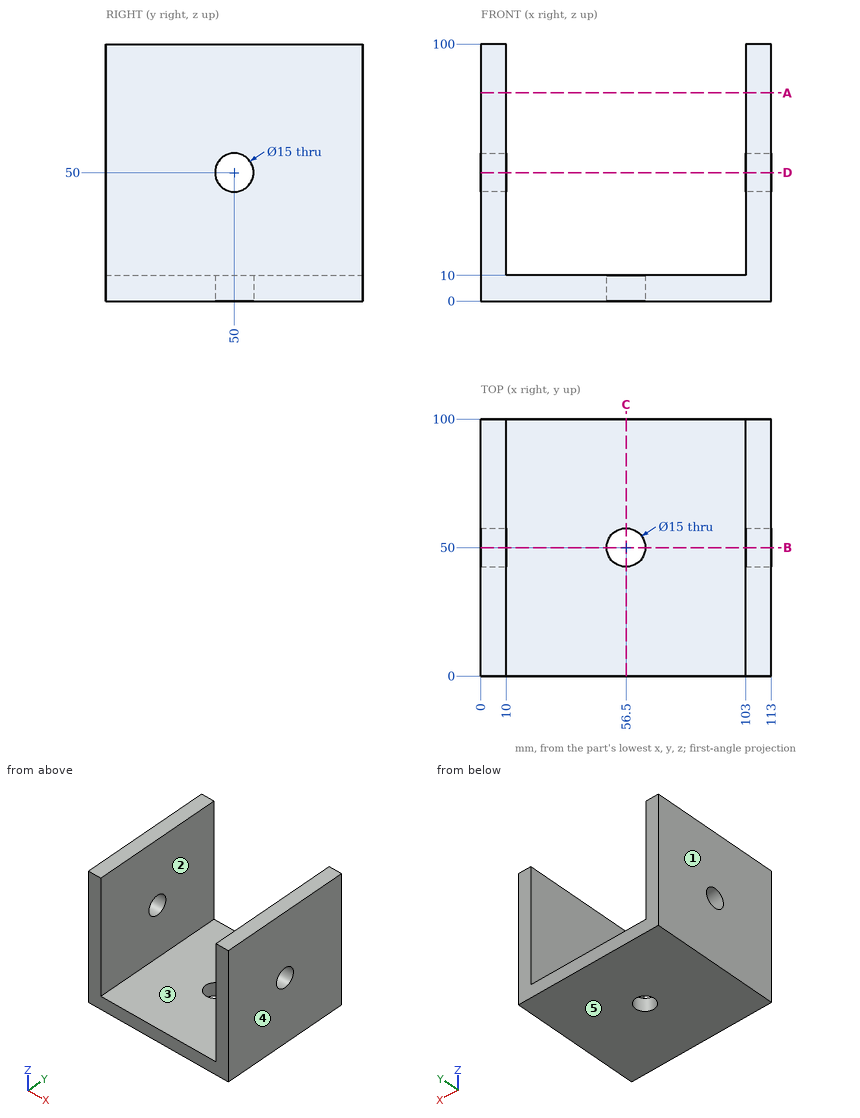
Print and shaded views of the part. All mm, measured from the part's lowest x, y and z. A direction names the side the tool comes from. Give positions to 0.01 mm unless a question says otherwise; leave off trailing zeros. Order: outer loops, then holes, each group sorted by start corner. A loop starts at its lowest first (then second) coordinate and runs counter-clockwise, first axis right, second up. Notation, with made-up numbers: (-23, 36) -> (7, 36) arc R15 ccw to (7, 47) -> close; hole circle Ø9 at (26, 79). An arc over 180 degrees is marked (long way). Use CSV: the item, a comma, the result in double quotes.
1. Drill centre lines: line 1 along Y through (x, z) = (56, 3); line 2 along X through (y, z) = (17, 78); line 3 along Z through (x, y) = (84.5, 13). Where is each one in solid material? Low to high. Write a range as from..to.
Outcome:
line 1,"0..42.52, 57.48..100"
line 2,"0..10, 103..113"
line 3,"0..10"
2. Band-saw the part on A-A, the plane z = 81. Give the cut face in (x, y).
Outcome:
outline,"(0, 0) -> (10, 0) -> (10, 100) -> (0, 100) -> close; (103, 0) -> (113, 0) -> (113, 100) -> (103, 100) -> close"
3. Band-saw the part on B-B, the plane y = 50. Give the cut face in (x, z).
Outcome:
outline,"(0, 0) -> (49, 0) -> (49, 10) -> (10, 10) -> (10, 42.5) -> (0, 42.5) -> close; (0, 57.5) -> (10, 57.5) -> (10, 100) -> (0, 100) -> close; (64, 0) -> (113, 0) -> (113, 42.5) -> (103, 42.5) -> (103, 10) -> (64, 10) -> close; (103, 57.5) -> (113, 57.5) -> (113, 100) -> (103, 100) -> close"
4. Band-saw the part on D-D, the plane z = 50. Give the cut face in (x, y).
Outcome:
outline,"(0, 0) -> (10, 0) -> (10, 42.5) -> (0, 42.5) -> close; (0, 57.5) -> (10, 57.5) -> (10, 100) -> (0, 100) -> close; (103, 0) -> (113, 0) -> (113, 42.5) -> (103, 42.5) -> close; (103, 57.5) -> (113, 57.5) -> (113, 100) -> (103, 100) -> close"
5. 3-axis set-ups, long thin cutter, end or side, ignore diameter. For the marked faces 1 and 2: which of +Z, -Z, +X, -X, +Y, -Y reach the whole face in a straight line?
Outcome:
face 1,"+Z, -Z, -X, +Y, -Y"
face 2,"+Z, +Y, -Y"
6. Mould opens along X. For the marked faces 3, 4 and 5 say: +X half, -X half, draft (parallel to the pull), parting line (faces both ways), or undercut.
Outcome:
face 3,"undercut"
face 4,"+X half"
face 5,"draft"
7. Band-saw the part on C-C, the plane x = 56.5. Give the cut face in (y, z).
Outcome:
outline,"(0, 0) -> (42.5, 0) -> (42.5, 10) -> (0, 10) -> close; (57.5, 0) -> (100, 0) -> (100, 10) -> (57.5, 10) -> close"
8. Drop a flat-ended pin along its axis: pin 1 (8 mm diameter, centred on x = 59.5, y = 34, fed in from +Z). Give the stop position or say it passes through.
Outcome:
pin 1,"z = 10"
